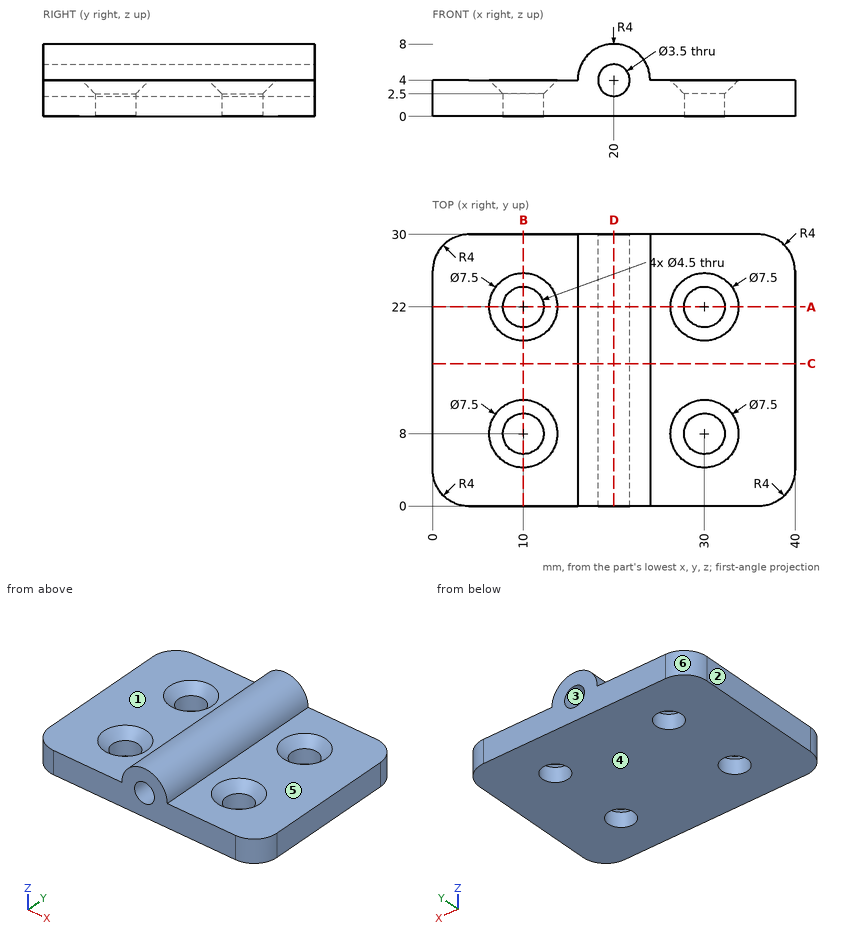
Can you work these out from the drawing? Everything is in mm from the part's minimum corner. A direction names the side the tool comes from. Give positions to 0.01 mm unless a question says otherwise; leave off trailing zeros. Loops run counter-clockwise (first coordinate to the right, second up) from the corner with the lowest first, then second, coordinate; pieces in that order, holes last. Notation, with made-up numbers: (-24, 71.5) - (-10, 71.5) arc R15 cw to (-10, 78.5) - close; hole circle Ø7 at (-33, 54). An arc over 180 degrees is marked (long way). Use one line per item in the form item = value.
1. I need wall thicknesses on probe 1 along X at (y, z) = (8, 0.85); probe 2 along Y at (x, z) = (10, 1.5); probe 3 along Z at (x, y) = (20, 16). Which ranges of each line are inside material? Lowest first, please.
Response values:
probe_1 = 0 to 7.75, 12.25 to 27.75, 32.25 to 40
probe_2 = 0 to 5.75, 10.25 to 19.75, 24.25 to 30
probe_3 = 0 to 2.25, 5.75 to 8
2. I want a section at D-D (x = 20). Please give me the cut outline in (y, z), and give its area (3 significant figures).
Response values:
outline = (0, 0) - (30, 0) - (30, 2.25) - (0, 2.25) - close; (0, 5.75) - (30, 5.75) - (30, 8) - (0, 8) - close
area = 135 mm²
3. I want a section at A-A (y = 22). Please give me the cut outline in (x, z).
Response values:
outline = (0, 0) - (7.75, 0) - (7.75, 2.5) - (6.25, 4) - (0, 4) - close; (12.25, 0) - (27.75, 0) - (27.75, 2.5) - (26.25, 4) - (24, 4) arc R4 ccw to (16, 4) - (13.75, 4) - (12.25, 2.5) - close; (32.25, 0) - (40, 0) - (40, 4) - (33.75, 4) - (32.25, 2.5) - close; hole circle Ø3.5 at (20, 4)
4. I want a section at C-C (y = 15.75). Please give me the cut outline in (x, z), and give its area (3 significant figures).
Response values:
outline = (0, 0) - (40, 0) - (40, 4) - (24, 4) arc R4 ccw to (16, 4) - (0, 4) - close; hole circle Ø3.5 at (20, 4)
area = 176 mm²
5. I want a section at B-B (x = 10). Please give me the cut outline in (y, z).
Response values:
outline = (0, 0) - (5.75, 0) - (5.75, 2.5) - (4.25, 4) - (0, 4) - close; (10.25, 0) - (19.75, 0) - (19.75, 2.5) - (18.25, 4) - (11.75, 4) - (10.25, 2.5) - close; (24.25, 0) - (30, 0) - (30, 4) - (25.75, 4) - (24.25, 2.5) - close
6. Thinking about a two-plate mould opening in Z: for the marked faces 3, 4, 5 and 6, which applies, released by +Z, released by -Z, zero draft, split by the parting line, or undercut?
Response values:
face_3 = undercut
face_4 = released by -Z
face_5 = released by +Z
face_6 = zero draft
7. I'm going to push flat-ended pins straight in: pin 1 Ø3.5 at (x, y) = (10, 22) entering from +Z; pin 2 Ø13 at (x, y) = (6, 15) entering from +Z; pin 3 Ø7 at (x, y) = (10, 8) entering from -Z; pin 4 Ø2 at (y, z) = (7.5, 6.5) entering from +X. Where does each tip first touch, or does it pass through?
Response values:
pin_1 = through
pin_2 = 4
pin_3 = 0
pin_4 = 23.71
8. On a 3-axis mill with a long thin cutter (end or side, diameter ignored), from which of +Z, -Z, +X, -X, +Y, -Y can I reach the whole of each face in a straight line? I mean the marked faces 1 and 2. Say none if no direction works.
Response values:
face_1 = +Z, -X, +Y, -Y
face_2 = +Z, -Z, -X, +Y, -Y
